Verification items for the finished model (mm, model axes). A direction names the side the tool comes from. Coordinates: 2 decimals unless noted, no trailing zeros. Loops run counter-clockwise (first coordinate to the right, second up) from the corner with the lowest first, then second, coordinate; pieces in that order, holes last. Notation, with made-up numbers: (0.5, 0) -> (19.5, 0) arc R19 cw to (19.5, 5) -> close; hole circle Ø4 at (7.5, -8). An arc over 180 degrees is marked (long way). Answer as a JSON object with one key per item and string values. Group by question number.
Q1. Scan lines: L1, parallel to Y at x = -1, z = 0.25; L2, parallel to Y at x = 20.5, z = 2.3. Record each from-to range of solid material in increasing order.
Q2. Release check for a two-part mould opening along X. For faces 1 (the flat face through (-22.225, 30, 2)), 2 (the flat face through (0, 0, 2.972)), 3 (the flat face through (31.75, 0, 1)), 4 (the flat face through (-9.525, 30, 2)) record: released by +X, released by -X, zero draft, split by the parting line, or undercut.
Q3. Set-up check for faces 5 (the flat face through (-27, 31.75, 1)), 6 (the flat face through (16, 28.778, 2)), 7 (the flat face through (-9.525, -30, 2)): record each of +Z, -Z, +X, -X, +Y, -Y from which the full face is reachable in a straight line by a thin tool's end or side.
Q4. Gauge pin test, flat end, axial feed: pin 1 Ø1.5 at (x, z) = (-17, 1.5) entering from -Y. Record the tip position at first contact, or that the pin passes through.
Q5. Cross-section at B-B on x = -18. Record the boundary of the cut face in (y, z), and give its area (3 significant figures).
```python
from build123d import *

# Parameters (mm, degrees)
SKETCH1_W           = 63.5
SKETCH1_H           = 63.5
BOSS_EXTRUDE1_DEPTH = 2.9718
SKETCH2_R           = 1.5875
SKETCH2_W           = 12.7
SKETCH2_H           = 2.9718
CUT_EXTRUDE1_DEPTH  = 45.999517722


with BuildPart() as part:
    # Sketch1 → Boss-Extrude1 (new body)
    with BuildSketch(Plane.XY):
        Rectangle(SKETCH1_W, SKETCH1_H)
    extrude(amount=BOSS_EXTRUDE1_DEPTH)

    # Sketch2 → Cut-Extrude1 (cut, through all)
    with BuildSketch(Plane.XY.offset(2.9718)):
        with Locations((0, -30.2641)):
            Circle(SKETCH2_R)
        with Locations((0, 30.2641)):
            Circle(SKETCH2_R)
        with Locations((15.875, -30.2641)):
            Rectangle(SKETCH2_W, SKETCH2_H)
        with Locations((-15.875, -30.2641)):
            Rectangle(SKETCH2_W, SKETCH2_H)
        with Locations((15.875, 30.2641)):
            Rectangle(SKETCH2_W, SKETCH2_H)
        with Locations((-15.875, 30.2641)):
            Rectangle(SKETCH2_W, SKETCH2_H)
    extrude(amount=-CUT_EXTRUDE1_DEPTH, mode=Mode.SUBTRACT)


solid = part.part
```
Computed values:
{
 "1": {"L1": "y = -31.75 to -31.5, -29.03 to 29.03, 31.5 to 31.75", "L2": "y = -28.78 to 28.78"},
 "2": {"face 1": "undercut", "face 2": "zero draft", "face 3": "released by +X", "face 4": "undercut"},
 "3": {"face 5": "+Z, -Z, +X, -X, +Y", "face 6": "+Z, -Z, +Y", "face 7": "+Z, -Z, -Y"},
 "4": {"pin 1": "stops at y = -28.78"},
 "5": {"outline": "(-28.78, 0) -> (28.78, 0) -> (28.78, 2.97) -> (-28.78, 2.97) -> close", "area": "171 mm²"}
}
